```python
from build123d import *

# Parameters (mm, degrees)
SKETCH_1_W               = 150
SKETCH_1_H               = 231
EXTRUDE_1_DEPTH          = 12.5
CUT_EXTRUDE_1_DEPTH      = 10.5
SKETCH_4_R               = 2.2
CUT_EXTRUDE_3_DEPTH      = 1
CUT_EXTRUDE_3_DEPTH_BACK = 13.5
SKETCH_5_R               = 2.2
SKETCH_5_R_2             = 1.6
SKETCH_5_R_3             = 1.5
CUT_EXTRUDE_4_DEPTH      = 13.5
SKETCH_6_R               = 1.5
CUT_EXTRUDE_5_DEPTH      = 10
SKETCH_3_R               = 1.6
CUT_EXTRUDE_6_DEPTH      = 10
SKETCH_7_W               = 10
SKETCH_7_H               = 231
CUT_EXTRUDE_7_DEPTH      = 13.5
SKETCH_8_W               = 10
SKETCH_8_H               = 231
CUT_EXTRUDE_8_DEPTH      = 13.5
SKETCH_9_W               = 43
SKETCH_9_H               = 102
EXTRUDE_2_DEPTH          = 10.5
SKETCH_10_R              = 1.6
CUT_EXTRUDE_9_DEPTH      = 30
SKETCH_11_W              = 130
SKETCH_11_H              = 231
CUT_EXTRUDE_10_DEPTH     = 9.5


with BuildPart() as part:
    # ｽｹｯﾁ1 → ﾎﾞｽ - 押し出し1 (new body)
    with BuildSketch(Plane.XY):
        Rectangle(SKETCH_1_W, SKETCH_1_H)
    extrude(amount=EXTRUDE_1_DEPTH)

    # ｽｹｯﾁ2 → ｶｯﾄ - 押し出し1 (cut)
    with BuildSketch(Plane.XY.offset(12.5)):
        Polygon((0, 115.5), (21.5, 115.5), (21.5, 13.5), (-21.5, 13.5), (-21.5, 115.5), align=None)
    extrude(amount=-CUT_EXTRUDE_1_DEPTH, mode=Mode.SUBTRACT)

    # ｽｹｯﾁ4 → ｶｯﾄ - 押し出し3 (cut, two sides)
    with BuildSketch(Plane.XY.offset(12.5)) as cut_extrude_3_sk:
        with Locations((-49.73, 74.5)):
            Circle(SKETCH_4_R)
        with Locations((49.73, 74.5)):
            Circle(SKETCH_4_R)
    extrude(amount=CUT_EXTRUDE_3_DEPTH, mode=Mode.SUBTRACT)
    extrude(cut_extrude_3_sk.sketch, amount=-CUT_EXTRUDE_3_DEPTH_BACK, mode=Mode.SUBTRACT)

    # ｽｹｯﾁ5 → ｶｯﾄ - 押し出し4 (cut, through all)
    with BuildSketch(Plane.XY.offset(12.5)):
        with Locations((18.25, -85)):
            Circle(SKETCH_5_R)
        with Locations((18.25, -12.95)):
            Circle(SKETCH_5_R_2)
        with Locations((-41.75, -45.48)):
            Circle(SKETCH_5_R_3)
        with Locations((-31.45, -67.68)):
            Circle(SKETCH_5_R_3)
        with Locations((-18.25, -85)):
            Circle(SKETCH_5_R)
        with Locations((-18.25, -12.95)):
            Circle(SKETCH_5_R_2)
        with Locations((0, -105.5)):
            Circle(SKETCH_5_R)
        with Locations((-59.34, -105.5)):
            Circle(SKETCH_5_R_3)
        with Locations((-37.14, -95.2)):
            Circle(SKETCH_5_R_3)
    extrude(amount=-CUT_EXTRUDE_4_DEPTH, mode=Mode.SUBTRACT)

    # ｽｹｯﾁ6 → ｶｯﾄ - 押し出し5 (cut)
    with BuildSketch(Plane.XY.offset(2)):
        with Locations((-12.5, 105.5)):
            Circle(SKETCH_6_R)
        with Locations((12.5, 105.5)):
            Circle(SKETCH_6_R)
    extrude(amount=-CUT_EXTRUDE_5_DEPTH, mode=Mode.SUBTRACT)

    # ｽｹｯﾁ3 → ｶｯﾄ - 押し出し6 (cut)
    with BuildSketch(Plane.XY.offset(2)):
        with Locations((-16.23, 42.5)):
            Circle(SKETCH_3_R)
        with Locations((16.23, 42.5)):
            Circle(SKETCH_3_R)
        with Locations((-16.23, 24.1)):
            Circle(SKETCH_3_R)
        with Locations((16.23, 24.1)):
            Circle(SKETCH_3_R)
    extrude(amount=-CUT_EXTRUDE_6_DEPTH, mode=Mode.SUBTRACT)

    # ｽｹｯﾁ7 → ｶｯﾄ - 押し出し7 (cut, through all)
    with BuildSketch(Plane.XY.offset(12.5)):
        with Locations((-70, 0)):
            Rectangle(SKETCH_7_W, SKETCH_7_H)
    extrude(amount=-CUT_EXTRUDE_7_DEPTH, mode=Mode.SUBTRACT)

    # ｽｹｯﾁ8 → ｶｯﾄ - 押し出し8 (cut, through all)
    with BuildSketch(Plane.XY.offset(12.5)):
        with Locations((70, 0)):
            Rectangle(SKETCH_8_W, SKETCH_8_H)
    extrude(amount=-CUT_EXTRUDE_8_DEPTH, mode=Mode.SUBTRACT)

    # ｽｹｯﾁ9 → ﾎﾞｽ - 押し出し2 (add)
    with BuildSketch(Plane.XY.offset(2)):
        with Locations((0, 64.5)):
            Rectangle(SKETCH_9_W, SKETCH_9_H)
    extrude(amount=EXTRUDE_2_DEPTH)

    # ｽｹｯﾁ10 → ｶｯﾄ - 押し出し9 (cut)
    with BuildSketch(Plane(origin=(0, 0, 0), x_dir=(-1, 0, 0), z_dir=(0, 0, -1))):
        with Locations((-16.23, 24.1)):
            Circle(SKETCH_10_R)
        with Locations((-16.23, 42.5)):
            Circle(SKETCH_10_R)
        with Locations((16.23, 42.5)):
            Circle(SKETCH_10_R)
        with Locations((16.23, 24.1)):
            Circle(SKETCH_10_R)
    extrude(amount=-CUT_EXTRUDE_9_DEPTH, mode=Mode.SUBTRACT)

    # ｽｹｯﾁ11 → ｶｯﾄ - 押し出し10 (cut)
    with BuildSketch(Plane.XY.offset(12.5)):
        Rectangle(SKETCH_11_W, SKETCH_11_H)
    extrude(amount=-CUT_EXTRUDE_10_DEPTH, mode=Mode.SUBTRACT)


solid = part.part
```
Check sheet for the modelled part. Datum: model origin and axes. Units: mm. Round coordinates to 2 decimals unless told otherwise and drop trailing zeros. Order: outer loops, then holes, each group sorted by start corner. A loop starts at its lowest first (then second) coordinate and runs counter-clockwise, first axis right, second up. Notation, with made-up numbers: (60, -36.5) -> (80, -36.5) arc R20 ccw to (80, -25.5) -> close; hole circle Ø8 at (64.25, -39.5). An arc over 180 degrees is marked (long way). One line per item, written item: value. Start each with the question number.
Q1. Cross-section at A-A (x = 49.73). Record the boundary of the cut face in (y, z), and give its area (3 significant figures).
Q2. Mould release check, pull along X, two halves, no side actions. Record for faces 1 (the face through (1.183, -103.645, 1.521)), 2 (the face through (-1, 2, 0)): pulls with the +X half, pulls with the -X half, needs draft (parallel to the pull), parting line crosses it, or undercut.
Q3. Thickness scan on line 1 (X direction, y = 105.5, z = 0.5); line 2 (Y direction, x = -18.25, z = 1.4); line 3 (Y direction, x = 0, z = 1.1). Record the ranges inside material, lowest first.
Completed:
1. outline: (-115.5, 0) -> (72.3, 0) -> (72.3, 3) -> (-115.5, 3) -> close; (76.7, 0) -> (115.5, 0) -> (115.5, 3) -> (76.7, 3) -> close
1. area: 680 mm²
2. face 1: undercut
2. face 2: needs draft
3. line 1: x = -65 to -14, -11 to 11, 14 to 65
3. line 2: y = -115.5 to -87.2, -82.8 to -14.55, -11.35 to 115.5
3. line 3: y = -115.5 to -107.7, -103.3 to 115.5
